Can you work these out from the model? Positions are in its coordinate system, mm. A direction names the side the tool comes from. Give positions to 0.01 mm unless a question says otherwise; leave off trailing zeros. Loops run counter-clockwise (first coordinate to the right, second up) from the corner with the lowest first, then second, coordinate; pieces in that order, holes last. Notation, with made-up numbers: (1.25, 64.25) - (23.25, 64.25) arc R21 ccw to (23.25, 76.25) - close; hole circle Ø1 at (33, 36.5). An arc over 180 degrees is marked (long way). Answer in a Markdown table with one row per item.
from build123d import *

# Parameters (mm, degrees)
ESQUISSE1_R             = 75
BOSS_EXTRU_1_DEPTH      = 105
BOSS_EXTRU_1_DEPTH_BACK = 105
BOSS_EXTRU_2_DEPTH      = 20
BOSS_EXTRU_2_DEPTH_BACK = 20
ESQUISSE1_4_R           = 75
BOSS_EXTRU_3_DEPTH      = 140
BOSS_EXTRU_3_DEPTH_BACK = 140


with BuildPart() as part:
    # Esquisse1 → Boss.-Extru.1 (new body, two sides)
    with BuildSketch(Plane.XY) as boss_extru_1_sk:
        Polygon((0, 0), (65, 0), (100.963541268, 34.939277283), (189.435353132, 52.357657653), (327.774435506, 318.557391477), (194.674568594, 387.726932664), (103.646308232, 282.906907711), (100.963541268, 268.22841359), (139.16368684, 248.376503864), (123.528365835, 180.14501013), (54.931728108, 221.309330755), (-15.068271892, 221.309330755), (-60.266641359, 189.970737975), (-93.12076123, 122.549622532), (-68.596637727, 41.164320625), align=None)
        with Locations((10.953732474, 122.549622532)):
            Circle(ESQUISSE1_R, mode=Mode.SUBTRACT)
    extrude(amount=BOSS_EXTRU_1_DEPTH)
    extrude(boss_extru_1_sk.sketch, amount=-BOSS_EXTRU_1_DEPTH_BACK)

    # Esquisse1_3 → Boss.-Extru.2 (add, two sides)
    with BuildSketch(Plane.XY) as boss_extru_2_sk:
        Polygon((189.435353132, 0), (65, 0), (100.963541268, 34.939277283), (189.435353132, 52.357657653), align=None)
    extrude(amount=BOSS_EXTRU_2_DEPTH)
    extrude(boss_extru_2_sk.sketch, amount=-BOSS_EXTRU_2_DEPTH_BACK)

    # Esquisse1_4 → Boss.-Extru.3 (add, two sides)
    with BuildSketch(Plane.XY) as boss_extru_3_sk:
        with Locations((10.953732474, 122.549622532)):
            Circle(ESQUISSE1_4_R)
    extrude(amount=BOSS_EXTRU_3_DEPTH)
    extrude(boss_extru_3_sk.sketch, amount=-BOSS_EXTRU_3_DEPTH_BACK)


solid = part.part
Q1. Imagine slicing it at A-A, the plane z = -73. Write out the boundary of the cut face in (x, y), and give its area (3 significant figures).
Checked values:
| item | result |
|---|---|
| outline | (-93.12, 122.55) - (-68.6, 41.16) - (0, 0) - (65, 0) - (100.96, 34.94) - (189.44, 52.36) - (327.77, 318.56) - (194.67, 387.73) - (103.65, 282.91) - (100.96, 268.23) - (139.16, 248.38) - (123.53, 180.15) - (54.93, 221.31) - (-15.07, 221.31) - (-60.27, 189.97) - close |
| area | 81,900 mm² |
Q2. Imagine slicing it at B-B, the plane y = 71.5. Write out the boundary of the cut face in (x, z), and give its area (3 significant figures).
Checked values:
| item | result |
|---|---|
| outline | (-77.74, -105) - (-43.99, -105) - (-43.99, -140) - (65.9, -140) - (65.9, -105) - (199.38, -105) - (199.38, 105) - (65.9, 105) - (65.9, 140) - (-43.99, 140) - (-43.99, 105) - (-77.74, 105) - close |
| area | 65,900 mm² |
Q3. For pin 1 (4 mm diameter, centred on x = 190.5, z = -35, fed in from +Y); pin 2 (2 mm diameter, centred on y = 76.5, z = -7, fed in from +X); pin 3 (10 mm diameter, centred on y = 339, z = -3, fed in from +X), each with a flat end and sliding along its axis, tell me the tip position at first contact or that it passes through.
Checked values:
| item | result |
|---|---|
| pin 1 | stops at y = 385.22 |
| pin 2 | stops at x = 202.5 |
| pin 3 | stops at x = 298.06 |
Q4. Imagine slicing it at C-C, the plane x = 9.5. Write out the boundary of the cut face in (y, z).
Checked values:
| item | result |
|---|---|
| outline | (0, -105) - (47.56, -105) - (47.56, -140) - (197.54, -140) - (197.54, -105) - (221.31, -105) - (221.31, 105) - (197.54, 105) - (197.54, 140) - (47.56, 140) - (47.56, 105) - (0, 105) - close |
Q5. If I drill on line 1 (X direction, y = 189, z = -6); line 2 (Y direction, x = 33, z = 67); line 3 (Z direction, x = 5, y = 28.5), over which ranges is the centre line in solid material (lowest first)? Write a range as [from, to].
Checked values:
| item | result |
|---|---|
| line 1 | x = [-60.74, 108.77], [125.56, 260.45] |
| line 2 | y = [0, 221.31] |
| line 3 | z = [-105, 105] |
Q6. On a 3-axis mill with a long thin cutter (end or side, diameter ignored), from which of +Z, -Z, +X, -X, +Y, -Y can I reach the whole of each face in a straight line? I mean faces 1 (the face through (142, 21, 20)), 2 (the face through (10, 124, 140)), 3 (the face through (82.73, 17.225, -61.905)), 4 (the face through (20, 221.309, 1)), 5 (the face through (119.8, 258.44, 1.47)). Say none if no direction works.
Checked values:
| item | result |
|---|---|
| face 1 | +Z, +X, -Y |
| face 2 | +Z, +X, -X, +Y, -Y |
| face 3 | -Z, +X, -Y |
| face 4 | +Z, -Z, -X, +Y |
| face 5 | +Z, -Z, -X |
Q7. Imagine slicing it at D-D, the plane z = 2. Write out the boundary of the cut face in (x, y).
Checked values:
| item | result |
|---|---|
| outline | (-93.12, 122.55) - (-68.6, 41.16) - (0, 0) - (189.44, 0) - (189.44, 52.36) - (327.77, 318.56) - (194.67, 387.73) - (103.65, 282.91) - (100.96, 268.23) - (139.16, 248.38) - (123.53, 180.15) - (54.93, 221.31) - (-15.07, 221.31) - (-60.27, 189.97) - close |
Q8. If we mould it in two halves opening along Y, with no side actions, what happens to faces 6 (the face through (144.58, 43.527, -61.905)), 7 (the face through (189.435, 27, 0)), 8 (the face through (-37.35, 205.86, 1.47)), 9 (the face through (89.71, 200.44, 1.47))? For each: released by +Y, released by -Y, zero draft, split by the parting line, or undercut.
Checked values:
| item | result |
|---|---|
| face 6 | released by -Y |
| face 7 | zero draft |
| face 8 | released by +Y |
| face 9 | undercut |
